Verification items for this drawing (mm, ordinates from the low corner). Round coordinates to 2 decimals unless told otherwise and drop trailing zeros. Order: outer loops, then holes, each group sorted by start corner. A loop starts at its lowest first (then second) coordinate and runs counter-clockwise, first axis right, second up. Notation, with made-up numbers: M 18,15.5 L 39,15.5 A17 cw 39,22.5 Z; hole C 59,40 d11. An arc over 180 degrees is marked long. Return JSON: item names as keys, results as strings. Group by question number.
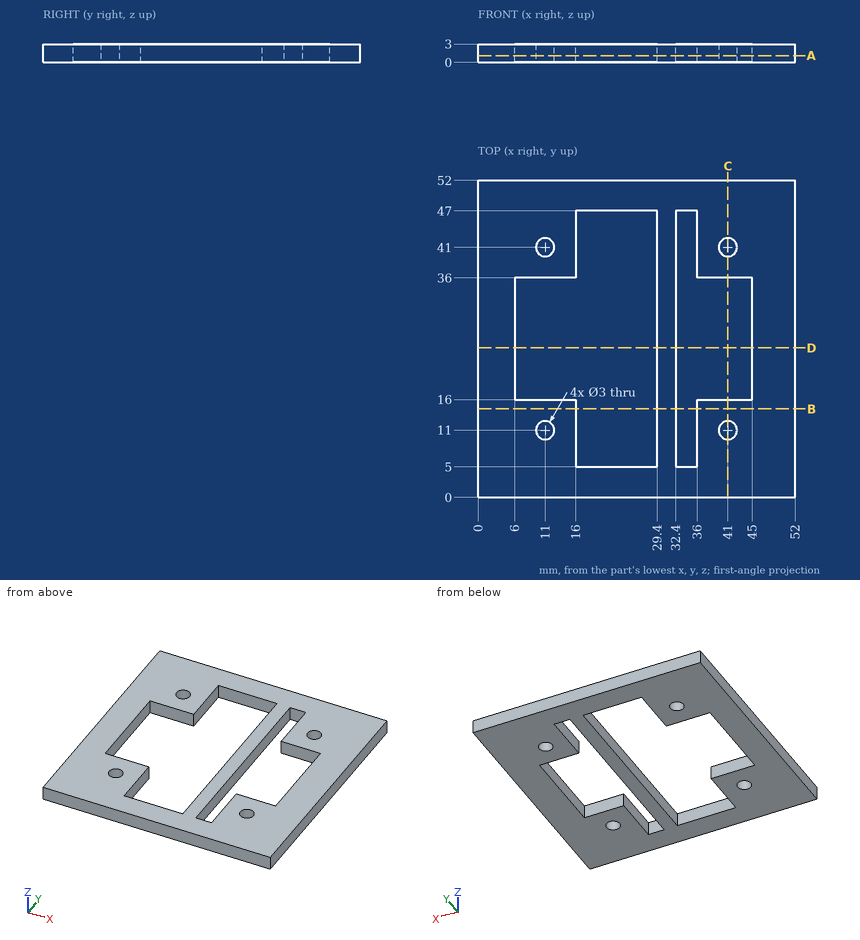
1. Cross-section at B-B (y = 14.5). Enter the section's corners in (x, z), plus the area to 3 significant figures.
2. Cross-section at A-A (z = 1.1). Enter the section's corners in (x, y), plus the area to 3 significant figures.
3. Cross-section at C-C (x = 41). Enter the section's corners in (y, z).
4. Cross-section at D-D (y = 24.5). Enter the section's corners in (x, z).
5. Go/stop test with flat-tipped pins: pin 1 (2 mm diameter, centred on x = 37, y = 10.5, fed in from -Z); pin 2 (2.5 mm diameter, centred on x = 11, y = 41, fed in from +Z). Record where each tip stops, or that it passes through.
6. Thickness scan on line 1 along X through (y, z) = (6, 2.55); line 2 along Y through (x, z) = (41, 1.7); line 3 along X through (y, z) = (41, 1.9). Record the ranges inside material, lowest first. Write a range as from..to.
Computed:
{
 "1": {"outline": "M 0,0 L 16,0 L 16,3 L 0,3 Z; M 29.4,0 L 32.4,0 L 32.4,3 L 29.4,3 Z; M 36,0 L 52,0 L 52,3 L 36,3 Z", "area": "105 mm²"},
 "2": {"outline": "M 0,0 L 52,0 L 52,52 L 0,52 Z; hole M 6,16 L 16,16 L 16,5 L 29.4,5 L 29.4,47 L 16,47 L 16,36 L 6,36 Z; hole C 11,11 d3; hole C 11,41 d3; hole M 32.4,5 L 36,5 L 36,16 L 45,16 L 45,36 L 36,36 L 36,47 L 32.4,47 Z; hole C 41,11 d3; hole C 41,41 d3", "area": "1,580 mm²"},
 "3": {"outline": "M 0,0 L 9.5,0 L 9.5,3 L 0,3 Z; M 12.5,0 L 16,0 L 16,3 L 12.5,3 Z; M 36,0 L 39.5,0 L 39.5,3 L 36,3 Z; M 42.5,0 L 52,0 L 52,3 L 42.5,3 Z"},
 "4": {"outline": "M 0,0 L 6,0 L 6,3 L 0,3 Z; M 29.4,0 L 32.4,0 L 32.4,3 L 29.4,3 Z; M 45,0 L 52,0 L 52,3 L 45,3 Z"},
 "5": {"pin 1": "stops at z = 0", "pin 2": "passes through"},
 "6": {"line 1": "x = 0..16, 29.4..32.4, 36..52", "line 2": "y = 0..9.5, 12.5..16, 36..39.5, 42.5..52", "line 3": "x = 0..9.5, 12.5..16, 29.4..32.4, 36..39.5, 42.5..52"}
}
